Could you check a few things on this model? Use its own coordinates, in mm. A direction names the side the tool comes from. Round coordinates to 2 decimals unless told otherwise and drop trailing zeros. Write each loop counter-clockwise with the first axis right and the second up, starting at its lowest first coordinate (ties: lowest second). Pieces come first, ordered by that corner, then holes. Notation, with made-up numbers: (57, 2.25) -> (66, 2.25) arc R25 cw to (66, 28.25) -> close; hole circle Ø8 at (0, 24.5). An arc over 180 degrees is marked (long way). Return JSON: item names as keys, results as strings.
from build123d import *

# Parameters (mm, degrees)
EXTRUDE_1_DEPTH          = 170
SKETCH_2_R               = 60
CUT_EXTRUDE_1_DEPTH      = 180
CUT_EXTRUDE_2_DEPTH      = 313.955268369
CUT_EXTRUDE_2_DEPTH_BACK = 313.955268369
SKETCH_3_R               = 11
FILLET_1_R               = 70
FILLET_2_R               = 5
FILLET_3_R               = 10
SKETCH_6_R               = 30
CUT_EXTRUDE_6_DEPTH      = 39
SKETCH_7_R               = 13
CUT_EXTRUDE_7_DEPTH      = 0.7
SKETCH_8_R               = 2.5
CUT_EXTRUDE_8_DEPTH      = 10
SKETCH_9_R               = 6
CUT_EXTRUDE_9_DEPTH      = 4
SKETCH_10_R              = 2.5
CUT_EXTRUDE_10_DEPTH     = 10
CUT_EXTRUDE_START        = -4
SKETCH_11_R              = 6
SKETCH_11_R_2            = 2.5
CUT_EXTRUDE_11_DEPTH     = 4
SKETCH_12_R              = 2.75
CUT_EXTRUDE_12_DEPTH     = 10


with BuildPart() as part:
    # 草图1 → 凸台-拉伸1 (new body)
    with BuildSketch(Plane.XY):
        Polygon((-180, 0), (0, 0), (0, -175), (8, -175), (8, 8), (-180, 8), (-188, 8), (-188, -175), (-180, -175), align=None)
    extrude(amount=EXTRUDE_1_DEPTH)

    # 草图2 → 切除-拉伸1 (cut)
    with BuildSketch(Plane(origin=(0, 8, 0), x_dir=(1, 0, 0), z_dir=(0, 1, 0))):
        with Locations(Location((-90, -85, 0), (0, 0, 180))):
            Circle(SKETCH_2_R)
    extrude(amount=-CUT_EXTRUDE_1_DEPTH, mode=Mode.SUBTRACT)

    # 草图3 → 切除-拉伸2 (cut, two sides: drawn at the far end of the back side and taken through both)
    with BuildSketch(Plane(origin=(8, 0, 0), x_dir=(0, 0, -1), z_dir=(1, 0, 0)).offset(-CUT_EXTRUDE_2_DEPTH_BACK)):
        with Locations(Location((-85, -95, 0), (0, 0, 90))):
            Circle(SKETCH_3_R)
    extrude(amount=CUT_EXTRUDE_2_DEPTH + CUT_EXTRUDE_2_DEPTH_BACK, mode=Mode.SUBTRACT)

    # 圆角1
    fillet_1_edges = [part.edges().sort_by_distance(p)[0] for p in [
        (4, -175, 0),
        (4, -175, 170),
        (-184, -175, 170),
        (-184, -175, 0),
    ]]
    fillet(fillet_1_edges, radius=FILLET_1_R)

    # 圆角2
    fillet_2_edges = [part.edges().sort_by_distance(p)[0] for p in [
        (0, 0, 85),
        (-180, 0, 85),
    ]]
    fillet(fillet_2_edges, radius=FILLET_2_R)

    # 圆角3
    fillet_3_edges = [part.edges().sort_by_distance(p)[0] for p in [
        (-188, 8, 85),
        (8, 8, 85),
    ]]
    fillet(fillet_3_edges, radius=FILLET_3_R)

    # 草图6 → 切除-拉伸6 (cut)
    with BuildSketch(Plane.ZY.offset(188)):
        with Locations(Location((85, -95, 0), (0, 0, 270))):
            Circle(SKETCH_6_R)
    extrude(amount=-CUT_EXTRUDE_6_DEPTH, mode=Mode.SUBTRACT)

    # 草图7 → 切除-拉伸7 (cut)
    with BuildSketch(Plane.ZY):
        with Locations(Location((85, -95, 0), (0, 0, 270))):
            Circle(SKETCH_7_R)
    extrude(amount=-CUT_EXTRUDE_7_DEPTH, mode=Mode.SUBTRACT)

    # 草图8 → 切除-拉伸8 (cut)
    with BuildSketch(Plane(origin=(8, 0, 0), x_dir=(0, 0, -1), z_dir=(1, 0, 0))):
        with Locations(Location((-55, -95, 0), (0, 0, 90))):
            Circle(SKETCH_8_R)
        with Locations(Location((-115, -95, 0), (0, 0, 90))):
            Circle(SKETCH_8_R)
    extrude(amount=-CUT_EXTRUDE_8_DEPTH, mode=Mode.SUBTRACT)

    # 草图9 → 切除-拉伸9 (cut)
    with BuildSketch(Plane(origin=(8, 0, 0), x_dir=(0, 0, -1), z_dir=(1, 0, 0))):
        with Locations(Location((-55, -95, 0), (0, 0, 90))):
            Circle(SKETCH_9_R)
        with Locations(Location((-115, -95, 0), (0, 0, 90))):
            Circle(SKETCH_9_R)
    extrude(amount=-CUT_EXTRUDE_9_DEPTH, mode=Mode.SUBTRACT)

    # 草图10 → 切除-拉伸10 (cut)
    with BuildSketch(Plane.XZ):
        with Locations(Location((-55.742253069, 158.674753309, 0), (0, 0, 270))):
            Circle(SKETCH_10_R)
        with Locations(Location((-32.485217492, 142.390001682, 0), (0, 0, 270))):
            Circle(SKETCH_10_R)
        with Locations(Location((-9.066918551, 92.169297536, 0), (0, 0, 270))):
            Circle(SKETCH_10_R)
        with Locations(Location((-11.541409366, 63.885738097, 0), (0, 0, 270))):
            Circle(SKETCH_10_R)
        with Locations(Location((-16.325246691, 50.742253069, 0), (0, 0, 270))):
            Circle(SKETCH_10_R)
        with Locations(Location((-32.609998318, 27.485217492, 0), (0, 0, 270))):
            Circle(SKETCH_10_R)
        with Locations(Location((-124.257746931, 11.325246691, 0), (0, 0, 270))):
            Circle(SKETCH_10_R)
        with Locations(Location((-147.514782508, 27.609998318, 0), (0, 0, 270))):
            Circle(SKETCH_10_R)
        with Locations(Location((-170.933081449, 77.830702464, 0), (0, 0, 270))):
            Circle(SKETCH_10_R)
        with Locations(Location((-168.458590634, 106.114261903, 0), (0, 0, 270))):
            Circle(SKETCH_10_R)
        with Locations(Location((-163.674753309, 119.257746931, 0), (0, 0, 270))):
            Circle(SKETCH_10_R)
        with Locations(Location((-147.390001682, 142.514782508, 0), (0, 0, 270))):
            Circle(SKETCH_10_R)
    extrude(amount=-CUT_EXTRUDE_10_DEPTH, mode=Mode.SUBTRACT)

    # 草图11 → 切除-拉伸11 (cut)
    # profile 1 of 12: a face of its own
    with BuildSketch(Plane(origin=(0, 8, 0), x_dir=(1, 0, 0), z_dir=(0, 1, 0)).offset(CUT_EXTRUDE_START)):
        with Locations(Location((-32.485217492, -142.390001682, 0), (0, 0, 180))):
            Circle(SKETCH_11_R)
        with Locations(Location((-32.485217492, -142.390001682, 0), (0, 0, 90))):
            Circle(SKETCH_11_R_2, mode=Mode.SUBTRACT)
    # profile 2 of 12: a face of its own
    with BuildSketch(Plane(origin=(0, 8, 0), x_dir=(1, 0, 0), z_dir=(0, 1, 0)).offset(CUT_EXTRUDE_START)):
        with Locations(Location((-55.742253069, -158.674753309, 0), (0, 0, 180))):
            Circle(SKETCH_11_R)
        with Locations(Location((-55.742253069, -158.674753309, 0), (0, 0, 90))):
            Circle(SKETCH_11_R_2, mode=Mode.SUBTRACT)
    # profile 3 of 12: a face of its own
    with BuildSketch(Plane(origin=(0, 8, 0), x_dir=(1, 0, 0), z_dir=(0, 1, 0)).offset(CUT_EXTRUDE_START)):
        with Locations(Location((-147.390001682, -142.514782508, 0), (0, 0, 180))):
            Circle(SKETCH_11_R)
        with Locations(Location((-147.390001682, -142.514782508, 0), (0, 0, 90))):
            Circle(SKETCH_11_R_2, mode=Mode.SUBTRACT)
    # profile 4 of 12: a face of its own
    with BuildSketch(Plane(origin=(0, 8, 0), x_dir=(1, 0, 0), z_dir=(0, 1, 0)).offset(CUT_EXTRUDE_START)):
        with Locations(Location((-163.674753309, -119.257746931, 0), (0, 0, 180))):
            Circle(SKETCH_11_R)
        with Locations(Location((-163.674753309, -119.257746931, 0), (0, 0, 90))):
            Circle(SKETCH_11_R_2, mode=Mode.SUBTRACT)
    # profile 5 of 12: a face of its own
    with BuildSketch(Plane(origin=(0, 8, 0), x_dir=(1, 0, 0), z_dir=(0, 1, 0)).offset(CUT_EXTRUDE_START)):
        with Locations(Location((-168.458590634, -106.114261903, 0), (0, 0, 180))):
            Circle(SKETCH_11_R)
        with Locations(Location((-168.458590634, -106.114261903, 0), (0, 0, 90))):
            Circle(SKETCH_11_R_2, mode=Mode.SUBTRACT)
    # profile 6 of 12: a face of its own
    with BuildSketch(Plane(origin=(0, 8, 0), x_dir=(1, 0, 0), z_dir=(0, 1, 0)).offset(CUT_EXTRUDE_START)):
        with Locations(Location((-170.933081449, -77.830702464, 0), (0, 0, 180))):
            Circle(SKETCH_11_R)
        with Locations(Location((-170.933081449, -77.830702464, 0), (0, 0, 90))):
            Circle(SKETCH_11_R_2, mode=Mode.SUBTRACT)
    # profile 7 of 12: a face of its own
    with BuildSketch(Plane(origin=(0, 8, 0), x_dir=(1, 0, 0), z_dir=(0, 1, 0)).offset(CUT_EXTRUDE_START)):
        with Locations(Location((-147.514782508, -27.609998318, 0), (0, 0, 180))):
            Circle(SKETCH_11_R)
        with Locations(Location((-147.514782508, -27.609998318, 0), (0, 0, 90))):
            Circle(SKETCH_11_R_2, mode=Mode.SUBTRACT)
    # profile 8 of 12: a face of its own
    with BuildSketch(Plane(origin=(0, 8, 0), x_dir=(1, 0, 0), z_dir=(0, 1, 0)).offset(CUT_EXTRUDE_START)):
        with Locations(Location((-124.257746931, -11.325246691, 0), (0, 0, 180))):
            Circle(SKETCH_11_R)
        with Locations(Location((-124.257746931, -11.325246691, 0), (0, 0, 90))):
            Circle(SKETCH_11_R_2, mode=Mode.SUBTRACT)
    # profile 9 of 12: a face of its own
    with BuildSketch(Plane(origin=(0, 8, 0), x_dir=(1, 0, 0), z_dir=(0, 1, 0)).offset(CUT_EXTRUDE_START)):
        with Locations(Location((-32.609998318, -27.485217492, 0), (0, 0, 180))):
            Circle(SKETCH_11_R)
        with Locations(Location((-32.609998318, -27.485217492, 0), (0, 0, 90))):
            Circle(SKETCH_11_R_2, mode=Mode.SUBTRACT)
    # profile 10 of 12: a face of its own
    with BuildSketch(Plane(origin=(0, 8, 0), x_dir=(1, 0, 0), z_dir=(0, 1, 0)).offset(CUT_EXTRUDE_START)):
        with Locations(Location((-16.325246691, -50.742253069, 0), (0, 0, 180))):
            Circle(SKETCH_11_R)
        with Locations(Location((-16.325246691, -50.742253069, 0), (0, 0, 90))):
            Circle(SKETCH_11_R_2, mode=Mode.SUBTRACT)
    # profile 11 of 12: a face of its own
    with BuildSketch(Plane(origin=(0, 8, 0), x_dir=(1, 0, 0), z_dir=(0, 1, 0)).offset(CUT_EXTRUDE_START)):
        with Locations(Location((-11.541409366, -63.885738097, 0), (0, 0, 180))):
            Circle(SKETCH_11_R)
        with Locations(Location((-11.541409366, -63.885738097, 0), (0, 0, 90))):
            Circle(SKETCH_11_R_2, mode=Mode.SUBTRACT)
    # profile 12 of 12: a face of its own
    with BuildSketch(Plane(origin=(0, 8, 0), x_dir=(1, 0, 0), z_dir=(0, 1, 0)).offset(CUT_EXTRUDE_START)):
        with Locations(Location((-9.066918551, -92.169297536, 0), (0, 0, 180))):
            Circle(SKETCH_11_R)
        with Locations(Location((-9.066918551, -92.169297536, 0), (0, 0, 90))):
            Circle(SKETCH_11_R_2, mode=Mode.SUBTRACT)
    extrude(amount=CUT_EXTRUDE_11_DEPTH, mode=Mode.SUBTRACT)

    # 草图12 → 切除-拉伸12 (cut)
    with BuildSketch(Plane.ZY.offset(188)):
        with Locations(Location((94.058666579, -128.80740392, 0), (0, 0, 270))):
            Circle(SKETCH_12_R)
        with Locations(Location((75.941333421, -128.80740392, 0), (0, 0, 270))):
            Circle(SKETCH_12_R)
        with Locations(Location((60.251262658, -119.748737342, 0), (0, 0, 270))):
            Circle(SKETCH_12_R)
        with Locations(Location((51.19259608, -104.058666579, 0), (0, 0, 270))):
            Circle(SKETCH_12_R)
        with Locations(Location((51.19259608, -85.941333421, 0), (0, 0, 270))):
            Circle(SKETCH_12_R)
        with Locations(Location((60.251262658, -70.251262658, 0), (0, 0, 270))):
            Circle(SKETCH_12_R)
        with Locations(Location((75.941333421, -61.19259608, 0), (0, 0, 270))):
            Circle(SKETCH_12_R)
        with Locations(Location((94.058666579, -61.19259608, 0), (0, 0, 270))):
            Circle(SKETCH_12_R)
        with Locations(Location((109.748737342, -70.251262658, 0), (0, 0, 270))):
            Circle(SKETCH_12_R)
        with Locations(Location((118.80740392, -85.941333421, 0), (0, 0, 270))):
            Circle(SKETCH_12_R)
        with Locations(Location((118.80740392, -104.058666579, 0), (0, 0, 270))):
            Circle(SKETCH_12_R)
        with Locations(Location((109.748737342, -119.748737342, 0), (0, 0, 270))):
            Circle(SKETCH_12_R)
    extrude(amount=-CUT_EXTRUDE_12_DEPTH, mode=Mode.SUBTRACT)


solid = part.part
1) Will these pins go through, and if not, where does the flat tip stop? pin 1 Ø15.5 at (x, z) = (-32.49, 142.39) entering from -Y; pin 2 Ø3.5 at (y, z) = (-119.75, 109.75) entering from -X; pin 3 Ø6 at (x, z) = (-13.5, 64.5) entering from +Y.
Return value:
{"pin 1": "y = 0", "pin 2": "x = 0", "pin 3": "y = 4"}
2) Thinking about a two-plate mould opening in Z: for faces 4 (the face through (-159.25, 5.97, 123.31)), 5 (the face through (-11.903, 5.972, 54.797)), 6 (the face through (-183.94, -153.95, 19.96)), 7 (the face through (-69, 8, 27)), which applies, pulls with the +Z half, pulls with the -Z half, needs draft (parallel to the pull), parting line crosses it, or undercut?
Return value:
{"face 4": "undercut", "face 5": "undercut", "face 6": "pulls with the -Z half", "face 7": "needs draft"}
3) I want a section at A-A, the plane x = -90. Please give me the cut outline in (y, z), and give its area (3 significant figures).
Return value:
{"outline": "(0, 0) -> (8, 0) -> (8, 25) -> (0, 25) -> close; (0, 145) -> (8, 145) -> (8, 170) -> (0, 170) -> close", "area": "400 mm²"}
4) I want a section at C-C, the plane z = 128. Please give me the cut outline in (x, y).
Return value:
{"outline": "(-188, -169.16) -> (-180, -169.16) -> (-180, -5) arc R5 cw to (-175, 0) -> (-131.84, 0) -> (-131.84, 8) -> (-178, 8) arc R10 ccw to (-188, -2) -> close; (-48.16, 0) -> (-5, 0) arc R5 cw to (0, -5) -> (0, -169.16) -> (8, -169.16) -> (8, -2) arc R10 ccw to (-2, 8) -> (-48.16, 8) -> close"}
5) For faces 1 (the face through (-184.06, -59.01, 74.27)), 2 (the face through (-176.476, 5.972, 75.533)), 3 (the face through (-98, 2, 170)), which set-ups out of +Z, -Z, +X, -X, +Y, -Y let a thin tool reach every point of the face, with its end or its side?
Return value:
{"face 1": "-X", "face 2": "+Y", "face 3": "+Z, +X, -X, +Y, -Y"}
6) If I drill on probe 1 along Z at (x, y) = (0.55, -95); probe 2 along Z at (x, y) = (6.95, -95); probe 3 along X at (y, z) = (-36.5, 158.5), over which ranges is the centre line in solid material (lowest first)? Write a range as [from, to].
Return value:
{"probe 1": "[0, 52.5], [57.5, 72], [98, 112.5], [117.5, 170]", "probe 2": "[0, 49], [61, 74], [96, 109], [121, 170]", "probe 3": "[-188, -180], [0, 8]"}
7) I want a section at B-B, the plane y = -8.5. Please give me the cut outline in (x, z), and give its area (3 significant figures).
Return value:
{"outline": "(-188, 0) -> (-180, 0) -> (-180, 170) -> (-188, 170) -> close; (0, 0) -> (8, 0) -> (8, 170) -> (0, 170) -> close", "area": "2,720 mm²"}
